from build123d import *

# Parameters (mm, degrees)
SKETCH1_W           = 12.192
SKETCH1_H           = 10.16
BOSS_EXTRUDE1_DEPTH = 7.874


with BuildPart() as part:
    # Sketch1 → Boss-Extrude1 (new body)
    with BuildSketch(Plane(origin=(0, 0, 0), x_dir=(1, 0, 0), z_dir=(0, 1, 0))):
        Rectangle(SKETCH1_W, SKETCH1_H)
    extrude(amount=-BOSS_EXTRUDE1_DEPTH)

    # Sketch2 → Revolve1 (revolve)
    with BuildSketch(Plane(origin=(0, 0, 0), x_dir=(0, 0, -1), z_dir=(1, 0, 0))):
        Polygon((0, 0), (3.429, 0), (3.429, 3.81), (3.175, 3.81), (3.175, 6.35), (2.54, 7.366), (2.54, 12.954), (0, 12.954), align=None)
    revolve(axis=Axis((0, 0, 0), (0, 1, 0)))


solid = part.part
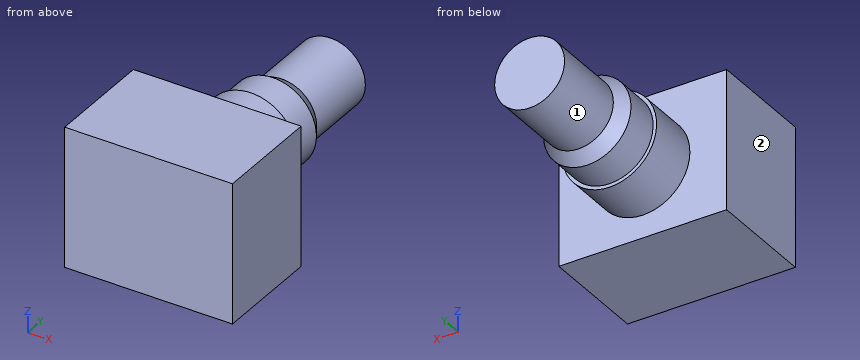
For this review, take the finished solid that the model builds, in its own axes (mm). Face numbers are marked on the shaded views. A direction names the side the tool comes from. Give positions to 0.01 mm unless a question says otherwise; leave off trailing zeros. Loops run counter-clockwise (first coordinate to the right, second up) from the corner with the lowest first, then second, coordinate; pieces in that order, holes last.
Item 1: For line 1 along Y through (x, z) = (-0.5, 4.25); line 2 along X through (y, z) = (6.25, -1); line 3 along Z through (x, y) = (-1.25, 0.5), list the stretches that pass through material, from the lowest coordinate up.
Item 2: Tool access review of the marked faces 1 and 2: name each direction out of +Z, -Z, +X, -X, +Y, -Y from which nothing blocks a thin tool from reaching the whole face with its end or side.
Item 3: Take a section at A-A, the plane x = 0. State the section outline as (y, z) points (3 decimals), and give its area (3 significant figures).
Item 4: Take a section at D-D, the plane x = -4.5. State the section outline as (y, z) points.
Item 5: Take a section at B-B, the plane z = 0. State the section outline as (x, y) points (3 decimals).
Item 6: Insertion check: pin 1 (2 mm diameter, centred on x = -2.5, y = 1.5, fed in from -Z); pin 2 (6 mm diameter, centred on y = 4.5, z = -3, fed in from +X). Each pin has a flat end and moves straight along its axis. Give the tip position at first contact, or say it passes through.
Item 7: Take a section at C-C, the plane y = 4.25. State the section outline as (x, z) points (3 decimals).
Calculated:
1. line 1: y = -7.87 to 0
1. line 2: x = -3.01 to 3.01
1. line 3: z = -3.19 to 3.19
2. face 1: +Y
2. face 2: +Z, -Z, -X, +Y, -Y
3. outline: (-7.874, -5.08) - (0, -5.08) - (0, -3.429) - (3.81, -3.429) - (3.81, -3.175) - (6.35, -3.175) - (7.366, -2.54) - (12.954, -2.54) - (12.954, 2.54) - (7.366, 2.54) - (6.35, 3.175) - (3.81, 3.175) - (3.81, 3.429) - (0, 3.429) - (0, 5.08) - (-7.874, 5.08) - close
3. area: 156 mm2
4. outline: (-7.87, -5.08) - (0, -5.08) - (0, 5.08) - (-7.87, 5.08) - close
5. outline: (-6.096, -7.874) - (6.096, -7.874) - (6.096, 0) - (3.429, 0) - (3.429, 3.81) - (3.175, 3.81) - (3.175, 6.35) - (2.54, 7.366) - (2.54, 12.954) - (-2.54, 12.954) - (-2.54, 7.366) - (-3.175, 6.35) - (-3.175, 3.81) - (-3.429, 3.81) - (-3.429, 0) - (-6.096, 0) - close
6. pin 1: stops at z = -3.08
6. pin 2: stops at x = 3.43
7. outline: circle Ø6.35 at (0, 0)
